Could you check a few things on this model? Use its own coordinates, in mm. A direction names the side the tool comes from. Give positions to 0.01 mm unless a question says otherwise; leave off trailing zeros. Write each loop counter-clockwise with the first axis right and the second up, starting at its lowest first coordinate (ties: lowest second). Pieces come first, ordered by that corner, then holes. Notation, with made-up numbers: (29, 53) - (48, 53) arc R23 ccw to (48, 79) - close; hole circle Ø10 at (68.25, 89). An arc over 180 degrees is marked (long way). Answer in a Markdown table with one row per item.
Autodesk Inventor part; units mm, degrees
ref_plane "Work Plane2" through (0, 0, 3) normal (0, 0, 1) x (1, 0, 0)
ref_plane "Work Plane8" through (0, 0, 0) normal (0.9238795, 0.3826834, 0) x (0, 0, 1)
ref_plane "Work Plane9" through (0, 0, 0) normal (1, 0, 0) x (0, 1, 0)
sketch "Sketch1" plane through (0, 0, 0) normal (0, 0, 1) x (1, 0, 0)
  circle A0 centre (0, 0) radius 2.5
  dimension "d0" = 5
extrude "Extrusion1" add sketch "Sketch1" along normal blind 6
ref_plane "Work Plane2" through (0, 0, 3) normal (0, 0, 1) x (1, 0, 0)
sketch "Sketch2" plane through (0, 0, 0) normal (0, 0, -1) x (-1, 0, 0)
  circle A0 centre (0, 0) radius 2.5
  circle A1 centre (0, 0) radius 2
  dimension "d3" = 4
surface extrude "ピッチ円直径" sketch "Sketch2" against normal through all shown no curves A1
ref_plane "Work Plane8" through (0, 0, 0) normal (0.9238795, 0.3826834, 0) x (0, 0, 1)
ref_plane "Work Plane9" through (0, 0, 0) normal (1, 0, 0) x (0, 1, 0)
spur gear teeth "平歯車" teeth 8 pitch diameter 4 tip diameter 5 root diameter 2.75 face width 6 start plane through (0, 0, 0) normal (0, 0, -1) x (-1, 0, 0)
sketch "スケッチ3" plane through (0, 0, 6) normal (0, 0, 1) x (1, 0, 0)
  point P0 (0, 0)
  point P1 (0, 0)
hole "穴1" at (0, 0, 6) direction (0, 0, -1) diameter 2 end through all
equation "\"d0\" = da_da"
equation "\"d1\" = da_b"
equation "\"d3\" = da_dw"
equation "\"d16\" = da_aw"
equation "\"d43\" = da_aw"
equation "\"d46\" = da_aw"
properties part number "平歯車1" material "アセタール樹脂、白"
1) If I drill on line 1 (Y direction, x = 0, z = 4.45); line 2 (Y direction, x = 1.65, z = 5.6), over which ranges is the centre line in solid material (lowest first)?
Check values:
| item | result |
|---|---|
| line 1 | y = -2.5 to -1, 1 to 2.5 |
| line 2 | y = -1.88 to -1.09, -0.42 to 0.42, 1.09 to 1.88 |
2) On a 3-axis mill with a long thin cutter (end or side, diameter ignored), from which of +Z, -Z, +X, -X, +Y, -Y can I reach the whole of each face in a straight line? I mean faces 1 (the face through (1.08, -1.64, 2.96)), 2 (the face through (-1.08, 1.64, 2.96)), 3 (the face through (1.9, -0.4, 3)). Say none if no direction works.
Check values:
| item | result |
|---|---|
| face 1 | +Z, -Z, -Y |
| face 2 | +Z, -Z, +Y |
| face 3 | +Z, -Z |
3) Imagine slicing it at D-D (y = -1.8). List the corners of the cut face in (x, z) for me.
Check values:
| item | result |
|---|---|
| outline | (-1.73, 0) - (-1.32, 0) - (-1.32, 6) - (-1.73, 6) - close; (-0.41, 0) - (0.41, 0) - (0.41, 6) - (-0.41, 6) - close; (1.32, 0) - (1.73, 0) - (1.73, 6) - (1.32, 6) - close |
4) Imagine slicing it at A-A (y = 0). List the corners of the cut face in (x, z) for me, then the cut area to 3 significant figures.
Check values:
| item | result |
|---|---|
| outline | (-2.5, 0) - (-1, 0) - (-1, 6) - (-2.5, 6) - close; (1, 0) - (2.5, 0) - (2.5, 6) - (1, 6) - close |
| area | 18.0 mm2 |
5) We'd pull the mould along X, two halves only. Please class faces 4 (the face through (-1.628, 1.064, 2.958)), 5 (the face through (0.4, -1.9, 3)), 6 (the face through (1.64, 1.08, 2.96)), 7 (the face through (1.064, 1.628, 2.958)): +X half, -X half, draft (parallel to the pull), parting line (faces both ways), or undercut.
Check values:
| item | result |
|---|---|
| face 4 | -X half |
| face 5 | undercut |
| face 6 | +X half |
| face 7 | undercut |
6) Will these pins go through, and if not, where does the flat tip stop? P1, Ø1.5, axis at x = -2, z = 0.5, coming from the -Y side; P2, Ø1, axis at y = 2, z = 4, coming from the -X side.
Check values:
| item | result |
|---|---|
| P1 | stops at y = -1.93 |
| P2 | stops at x = -1.93 |
